Could you check a few things on this drawing? It's one solid part, dimensions in mm from its lowest x, y, z. A direction names the side the tool comes from. Give positions to 0.01 mm unless a question says otherwise; leave off trailing zeros. Write each loop counter-clockwise with the first axis right and the second up, starting at its lowest first coordinate (ties: lowest second). Pieces come first, ordered by that corner, then holes. Notation, with made-up numbers: (53.5, 56.5) -> (83.5, 56.5) arc R9 ccw to (83.5, 60.5) -> close; hole circle Ø3 at (39, 70.5). An arc over 180 degrees is marked (long way). Use CSV: the item, a comma, the result in double quotes. Start each with the question number.
(1) Which directions (+Z, -Z, +X, -X, +Y, -Y) give clear straight access to the entire face, cutting with the end or side of a thin tool? Please do the marked faces 4, 5, 6 and 7.
(2) Suppose I cut it at D-D on z = 23.5. List the corners of the cut face in (x, y) for me.
(3) Suppose I cut it at B-B on z = 15.5. List the corners of the cut face in (x, y) for me.
(4) Suppose I cut it at C-C on y = 10. List the corners of the cut face in (x, z) for me, plus the area to 3 significant figures.
(5) For pin 1 Ø6 at (y, z) = (69.5, 33.5) entering from -X; pin 2 Ø22.5 at (y, z) = (63.5, 26) entering from -X; pin 3 Ø10 at (x, z) = (6.5, 6.5) entering from +Y; pin 4 Ø4 at (x, z) = (32, 29.5) entering from -Y, each with a flat end and sliding along its axis, tell me the tip position at first contact or that it passes through.
(6) If we mould it in two halves opening along X, with no side actions, what happens to the marked faces 1, 2 and 3? For each: pulls with the +X half, pulls with the -X half, needs draft (parallel to the pull), parting line crosses it, or undercut.
(7) Suppose I cut it at A-A on x = 14.5. List the corners of the cut face in (y, z) for me.
(8) I need wall thicknesses on L1, parallel to Z at x = 9, y = 55.5; L2, parallel to Y at x = 47, z = 38.5; L3, parallel to X at y = 31.5, z = 28. Which ranges of each line are inside material? Lowest first, please. Write a range as [from, to].
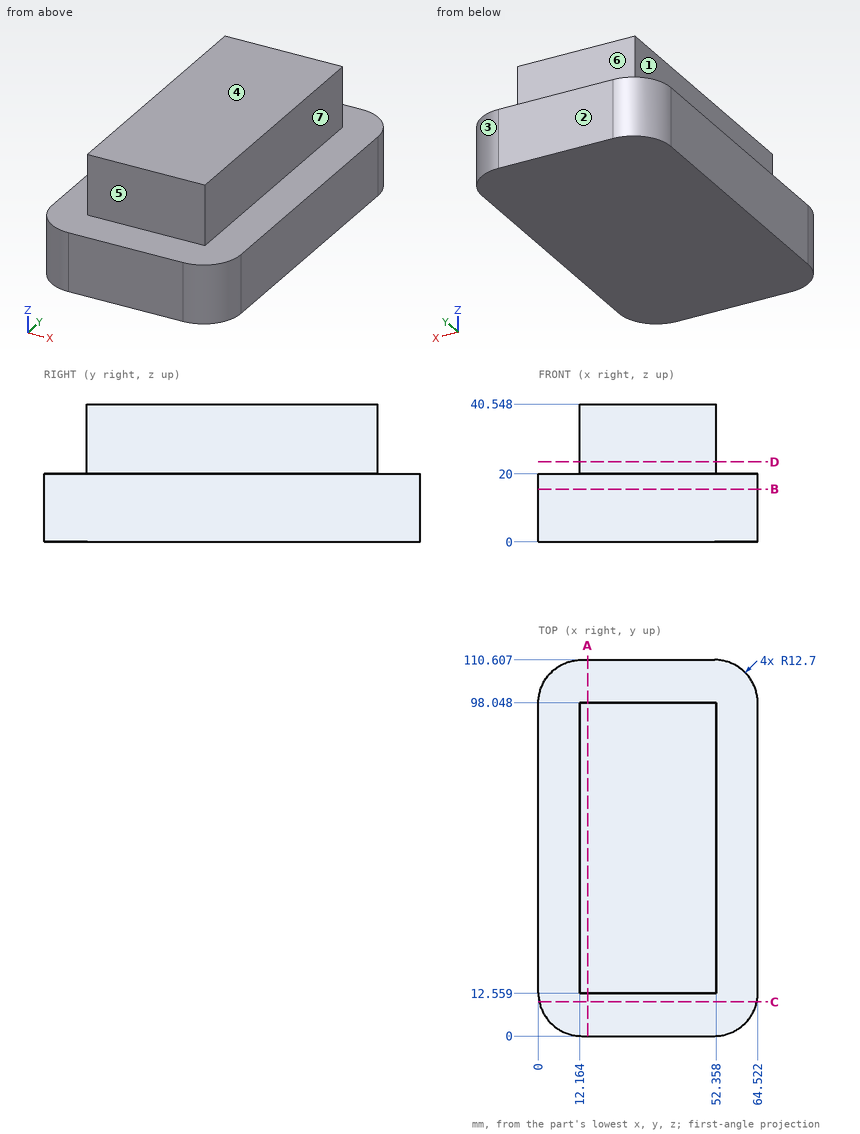
Geometry says:
1,face 4,"+Z, +X, -X, +Y, -Y"
1,face 5,"+Z, +X, -X, -Y"
1,face 6,"+Z, +X, -X, +Y"
1,face 7,"+Z, +X, +Y, -Y"
2,outline,"(12.16, 12.56) -> (52.36, 12.56) -> (52.36, 98.05) -> (12.16, 98.05) -> close"
3,outline,"(0, 12.7) arc R12.7 ccw to (12.7, 0) -> (51.82, 0) arc R12.7 ccw to (64.52, 12.7) -> (64.52, 97.91) arc R12.7 ccw to (51.82, 110.61) -> (12.7, 110.61) arc R12.7 ccw to (0, 97.91) -> close"
4,outline,"(0.29, 0) -> (64.23, 0) -> (64.23, 20) -> (0.29, 20) -> close"
4,area,"1,280 mm²"
5,pin 1,"x = 12.16"
5,pin 2,"x = 0"
5,pin 3,"y = 110.55"
5,pin 4,"y = 12.56"
6,face 1,"pulls with the -X half"
6,face 2,"needs draft"
6,face 3,"pulls with the +X half"
7,outline,"(0, 0) -> (110.61, 0) -> (110.61, 20) -> (98.05, 20) -> (98.05, 40.55) -> (12.56, 40.55) -> (12.56, 20) -> (0, 20) -> close"
8,L1,"[0, 20]"
8,L2,"[12.56, 98.05]"
8,L3,"[12.16, 52.36]"
